```python
from build123d import *

# Parameters (mm, degrees)
BOSS_EXTRUDE1_DEPTH = 6.35
FILLET1_R           = 5
SKETCH2_R           = 1.25
CUT_EXTRUDE1_DEPTH  = 20


with BuildPart() as part:
    # Sketch1 → Boss-Extrude1 (new body)
    with BuildSketch(Plane(origin=(0, 0, 0), x_dir=(1, 0, 0), z_dir=(0, 1, 0))):
        Polygon((-57.825, 26.738412941), (-42.825, 26.738412941), (-9.574489714, 0), (-42.825, -26.738412941), (-57.825, -26.738412941), (-57.825, -46.5), (-33.250510286, -46.5), (-33.250510286, -34.437743191), (0, -7.69933025), (33.250510286, -34.437743191), (33.250510286, -46.5), (57.825, -46.5), (57.825, -26.738412941), (42.825, -26.738412941), (9.574489714, 0), (42.825, 26.738412941), (57.825, 26.738412941), (57.825, 46.5), (33.250510286, 46.5), (33.250510286, 34.437743191), (0, 7.69933025), (-33.250510286, 34.437743191), (-33.250510286, 46.5), (-57.825, 46.5), align=None)
    extrude(amount=BOSS_EXTRUDE1_DEPTH)

    # Fillet1
    fillet1_edges = [part.edges().sort_by_distance(p)[0] for p in [
        (-33.250510286, 3.175, -34.437743191),
        (0, 3.175, -7.69933025),
        (33.250510286, 3.175, -34.437743191),
        (42.825, 3.175, -26.738412941),
        (9.574489714, 3.175, 0),
        (42.825, 3.175, 26.738412941),
        (33.250510286, 3.175, 34.437743191),
        (0, 3.175, 7.69933025),
        (-33.250510286, 3.175, 34.437743191),
        (-42.825, 3.175, 26.738412941),
        (-9.574489714, 3.175, 0),
    ]]
    fillet(fillet1_edges, radius=FILLET1_R)

    # Sketch2 → Cut-Extrude1 (cut)
    with BuildSketch(Plane(origin=(57.825, 0, 0), x_dir=(0, 0, -1), z_dir=(1, 0, 0))):
        with Locations((36.5, 3.175)):
            Circle(SKETCH2_R)
        with Locations(Location((-36.5, 3.175, 0), (0, 0, 180))):
            Circle(SKETCH2_R)
    cut_extrude1 = extrude(amount=-CUT_EXTRUDE1_DEPTH, mode=Mode.SUBTRACT)

    # Mirror1: Cut-Extrude1 across plane
    add(cut_extrude1.mirror(Plane(origin=(0, 0, 0), x_dir=(0, 0, 1), z_dir=(1, 0, 0))), mode=Mode.SUBTRACT)


solid = part.part
```
CAD build for the part. Positions are in the model's coordinates, mm. A direction names the side the tool comes from. Round coordinates to 2 decimals unless told otherwise and drop trailing zeros. Write each loop counter-clockwise with the first axis right and the second up, starting at its lowest first coordinate (ties: lowest second). Pieces come first, ordered by that corner, then holes.
Item 1: Tool access for faces 1 (the flat face through (33.251, 3, -42)), 2 (the cylindrical face through (-32.773, 3.219, 34.701)), 3 (the flat face through (28.13, 3.13, 14.92)): list every direction of +Z, -Z, +X, -X, +Y, -Y with a clear straight run to the whole face (end or side of a thin tool).
Filled in:
face 1: -Z, +Y, -Y
face 2: +Z, +Y, -Y
face 3: +X, +Y, -Y
Item 2: Band-saw the part on B-B on x = 50.5. Write the cut outline in (y, z) (3 decimals), then the cut area to 3 significant figures.
Filled in:
outline: (0, -46.5) - (6.35, -46.5) - (6.35, -26.738) - (0, -26.738) - close; (0, 26.738) - (6.35, 26.738) - (6.35, 46.5) - (0, 46.5) - close; hole circle Ø2.5 at (3.175, -36.5); hole circle Ø2.5 at (3.175, 36.5)
area: 241 mm2
Item 3: Drill centre lines: L1, parallel to Y at x = 48.5, z = -36.5 (3 decimals); L2, parallel to Z at x = -51.5, y = 2.75; L3, parallel to Z at x = -48, y = 3.75. Where is each one in solid material? Low to high.
Filled in:
L1: y = 0 to 1.925, 4.425 to 6.35
L2: z = -46.5 to -37.68, -35.32 to -26.74, 26.74 to 35.32, 37.68 to 46.5
L3: z = -46.5 to -37.61, -35.39 to -26.74, 26.74 to 35.39, 37.61 to 46.5
Item 4: Mould opens along X. For faces 4 (the cylindrical face through (-12.554, 3.219, -0.063)), 5 (the flat face through (-33.251, 3, 42)), 6 (the flat face through (0, 0, 7)), 7 (the cylindrical face through (12.554, 3.219, 0.063)) say: released by +X, released by -X, zero draft, split by the parting line, or undercut.
Filled in:
face 4: released by -X
face 5: undercut
face 6: zero draft
face 7: released by +X
Item 5: Band-saw the part on A-A on z = 39. Write the cut outline in (x, y) (3 decimals), then the cut area to 3 significant figures.
Filled in:
outline: (-57.825, 0) - (-33.251, 0) - (-33.251, 6.35) - (-57.825, 6.35) - close; (33.251, 0) - (57.825, 0) - (57.825, 6.35) - (33.251, 6.35) - close
area: 312 mm2
Item 6: Drop flat-ended pins along their axis: pin 1 Ø2 at (y, z) = (3.175, 36.5) entering from -X (3 decimals); pin 2 Ø0.8 at (y, z) = (3, 36.5) entering from +X (3 decimals). Give the stop position or say it passes through.
Filled in:
pin 1: stops at x = -37.825
pin 2: stops at x = 37.825
Item 7: Band-saw the part on C-C on z = -23. Write the cut outline in (x, y).
Filled in:
outline: (-38.18, 0) - (-19.03, 0) - (-19.03, 6.35) - (-38.18, 6.35) - close; (19.03, 0) - (38.18, 0) - (38.18, 6.35) - (19.03, 6.35) - close
